Read the model definition and answer for the solid it produces. Units are mm, in the model's axes. A direction names the side the tool comes from. Coordinates: 2 decimals unless noted, no trailing zeros.
```python
from build123d import *

# Parameters (mm, degrees)
F1_DEPTH = 7
F2_COUNT = 3


with BuildPart() as f1:
    # F0 (on Top) → F1 (new body)
    with BuildSketch(Plane.XY):
        with BuildLine():
            ThreePointArc((19.911619, -8.166607), (17.543738, -5.480184), (14.599963, -3.441086))
            ThreePointArc((14.599963, -3.441086), (12.370328, -8.483807), (8.469307, -12.38026))
            ThreePointArc((8.469307, -12.38026), (14.522507, -13.388086), (20.276548, -11.255493))
            ThreePointArc((20.276548, -11.255493), (29.817845, -9.18146), (29.413784, 0.574292))
            ThreePointArc((29.413784, 0.574292), (24.305689, 6.457834), (19.386908, 12.500541))
            ThreePointArc((19.386908, 12.500541), (18.899382, 14.842139), (20.276548, 16.79769))
            ThreePointArc((20.276548, 16.79769), (22.963658, 16.182674), (24.911437, 14.232043))
            ThreePointArc((24.911437, 14.232043), (27.294309, 13.34521), (28.733607, 15.441152))
            ThreePointArc((28.733607, 15.441152), (28.42968, 16.838907), (27.747044, 18.095927))
            ThreePointArc((27.747044, 18.095927), (27.819997, 18.82609), (28.394395, 19.282736))
            ThreePointArc((28.394395, 19.282736), (29.194592, 19.357364), (29.99479, 19.282736))
            ThreePointArc((29.99479, 19.282736), (31.313352, 20.013671), (32.350428, 21.107905))
            ThreePointArc((32.350428, 21.107905), (32.747453, 21.35798), (33.123679, 21.638373))
            ThreePointArc((33.123679, 21.638373), (33.236351, 21.937357), (33.215091, 22.256158))
            ThreePointArc((33.215091, 22.256158), (34.074746, 22.640916), (34.931641, 23.031782))
            ThreePointArc((34.931641, 23.031782), (35.395743, 23.023665), (35.859846, 23.031782))
            ThreePointArc((35.859846, 23.031782), (35.514758, 23.138271), (35.166871, 23.235226))
            ThreePointArc((35.166871, 23.235226), (35.408402, 23.631601), (35.497464, 24.087142))
            ThreePointArc((35.497464, 24.087142), (35.193756, 23.645558), (34.848992, 23.235226))
            ThreePointArc((34.848992, 23.235226), (33.969899, 22.894434), (33.123679, 22.478674))
            ThreePointArc((33.123679, 22.478674), (32.717605, 22.663576), (32.271761, 22.646023))
            ThreePointArc((32.271761, 22.646023), (31.722721, 22.59774), (31.17368, 22.646023))
            ThreePointArc((31.17368, 22.646023), (30.666364, 22.748602), (30.183258, 22.562858))
            ThreePointArc((30.183258, 22.562858), (29.515854, 22.463255), (28.849158, 22.359021))
            ThreePointArc((28.849158, 22.359021), (28.37224, 21.836259), (27.868547, 21.339245))
            ThreePointArc((27.868547, 21.339245), (26.616866, 20.751209), (25.524797, 19.902753))
            ThreePointArc((25.524797, 19.902753), (25.494877, 18.175258), (26.280845, 16.636625))
            ThreePointArc((26.280845, 16.636625), (26.333424, 16.296609), (26.008667, 16.182994))
            ThreePointArc((26.008667, 16.182994), (24.834884, 17.392019), (23.638841, 18.579029))
            ThreePointArc((23.638841, 18.579029), (19.553333, 19.540115), (16.213791, 16.997965))
            ThreePointArc((16.213791, 16.997965), (15.711707, 14.872374), (15.976911, 12.70445))
            ThreePointArc((15.976911, 12.70445), (21.162192, 3.810315), (27.695496, -4.146362))
            ThreePointArc((27.695496, -4.146362), (25.976142, -8.319526), (21.494055, -8.850903))
            ThreePointArc((21.494055, -8.850903), (22.328872, -2.938933), (17.131662, 0))
            ThreePointArc((17.131662, 0), (21.205283, -3.169777), (19.911619, -8.166607))
        make_face()
        with BuildLine():
            ThreePointArc((4.323353, -10.114772), (-9.180329, 6.059832), (11, 0))
            ThreePointArc((11, 0), (10.95098, -1.037323), (10.804357, -2.0654))
            ThreePointArc((10.804357, -2.0654), (12.749286, -2.62322), (14.599963, -3.441086))
            ThreePointArc((14.599963, -3.441086), (14.899655, -1.73213), (15, 0))
            ThreePointArc((15, 0), (-13.267245, 6.998586), (8.469307, -12.38026))
            ThreePointArc((8.469307, -12.38026), (8.380036, -12.339422), (8.291104, -12.29785))
            ThreePointArc((8.291104, -12.29785), (6.23471, -11.338114), (4.323353, -10.114772))
        make_face()
    extrude(amount=F1_DEPTH)

    # F2: F1 ×3 about axis
    f2_axis = Axis((0, 0, 0), (0, 0, -1))


with BuildPart() as f1_1:
    add(f1.part)
    for i in range(1, F2_COUNT):
        add(f1.part.rotate(f2_axis, i * 360 / F2_COUNT))


solid = f1_1.part
```
1) Which of the six approach directions +Z, -Z, +X, -X, +Y, -Y give full straight-line access (tool end or side, diameter ignored) to faces 1 (the cylindrical face through (2.62, -30.21, 3.45)), 2 (the cylindrical face through (-28.8, 16.2, 3.5)), 3 (the cylindrical face through (-1.304, -14.943, 3.451)), 4 (the cylindrical face through (-18.819, -5.804, 3.451))?
A:
face 1: +Z, -Z, +X
face 2: +Z, -Z, +Y
face 3: +Z, -Z
face 4: +Z, -Z, -X
2) Straight lines are drawn through the part: line 1 (X direction, y = -5.5, z = 0.5); line 2 (Y direction, x = -12.5, z = 2); line 3 (Y direction, x = -13, z = 4). For each, find the intervals that lie inside material, in ascending order.
A:
line 1: x = -18.67 to -9.53, 9.53 to 17.57, 21.38 to 22.87, 27.68 to 31.34
line 2: y = -25.41 to -20.89, -17.81 to -16.87, -12.07 to 8.29, 19.57 to 28.98
line 3: y = -25.51 to -20.97, -17.87 to -16.83, -12.27 to 7.48, 18.38 to 28.58
3) Flat-ended cylindrical pins translate along their axes: pin 1 Ø4 at (x, z) = (-22, 1) entering from -Y; pin 2 Ø10 at (x, y) = (-31, 9.5) entering from -Z; pin 3 Ø4 at (x, z) = (-25, 4.5) entering from +Y; pin 4 Ø1.5 at (x, z) = (-11.5, 4) entering from -Y. Find the tip coordinate at first contact, or state that the pin passes through.
A:
pin 1: stops at y = -24.7
pin 2: stops at z = 0
pin 3: stops at y = 17.51
pin 4: stops at y = -25.36
4) Determine the mould class of faces 5 (the cylindrical face through (28.437, 16.82, 3.451)), 6 (the cylindrical face through (-2.08, -30.27, 3.45)), 7 (the cylindrical face through (-4.59, 9.996, 3.451)) for opening direction X: pulls with the +X half, pulls with the -X half, needs draft (parallel to the pull), parting line crosses it, or undercut.
A:
face 5: pulls with the +X half
face 6: pulls with the -X half
face 7: undercut
